The listing builds one solid part. Answer for the finished solid, in the listing's coordinates (mm). A direction names the side the tool comes from. Coordinates: 2 decimals unless noted, no trailing zeros. Write each loop counter-clockwise with the first axis right and the second up, starting at its lowest first coordinate (ties: lowest second). Pieces come first, ordered by that corner, then holes. Notation, with made-up numbers: M 30.5,-31 L 64.5,-31 A22 cw 64.5,-25 Z; hole C 2,-10 d10. An arc over 180 degrees is marked long. Write item = value, one per line. Start each with the question number.
Solid Edge part; units mm, degrees
sketch "Sketch1" plane through (0, 0, 0) normal (0, 0, 1) x (1, 0, 0)
  line L0 (-10.25, -8) -> (10.25, -8)
  line L1 (10.25, -8) -> (10.25, 8)
  line L2 (10.25, 8) -> (-10.25, 8)
  line L3 (-10.25, 8) -> (-10.25, -8)
  dimension "D1" = 10.25
  dimension "D2" = 10.25
extrude "Protrusion1" add sketch "Sketch1" along normal blind 1.6
sketch "Sketch2" plane through (0, 0, 1.6) normal (0, 0, 1) x (1, 0, 0)
  circle A0 centre (-8, 5.8) radius 1.4
  circle A1 centre (8, 5.8) radius 1.4
extrude "Cutout1" cut sketch "Sketch2" against normal through all
sketch "Sketch3" plane through (0, 0, 1.6) normal (0, 0, 1) x (1, 0, 0)
  line L0 (-10.25, -3.5) -> (10.25, -3.5)
  line L1 (10.25, -3.5) -> (10.25, 4)
  line L2 (6.25, 4) -> (10.25, 4)
  line L3 (6.25, 5) -> (6.25, 4)
  line L4 (3.5, 5) -> (6.25, 5)
  line L5 (3.5, 8) -> (3.5, 5)
  line L6 (3.5, 8) -> (-3.5, 8)
  line L7 (-3.5, 8) -> (-3.5, 5)
  line L8 (-3.5, 5) -> (-6.25, 5)
  line L9 (-6.25, 5) -> (-6.25, 4)
  line L10 (-6.25, 4) -> (-10.25, 4)
  line L11 (-10.25, 4) -> (-10.25, -3.5)
  dimension "D1" = 3.5
  dimension "D2" = 3.5
  dimension "D3" = 10.25
  dimension "D4" = 6.25
  dimension "D5" = 10.25
  dimension "D6" = 3.5
  dimension "D7" = 6.25
extrude "Extrusionsausprägung_2" add sketch "Sketch3" along normal blind 1.5
sketch "Sketch4" plane through (0, -5.75, 1.6) normal (0, 0, 1) x (1, 0, 0)
  circle A0 centre (-8.75, -0.75) radius 0.5
  circle A1 centre (-6.25, -0.75) radius 0.5
  circle A2 centre (-3.75, -0.75) radius 0.5
  circle A3 centre (-1.25, -0.75) radius 0.5
  circle A4 centre (1.25, -0.75) radius 0.5
  circle A5 centre (3.75, -0.75) radius 0.5
  circle A6 centre (6.25, -0.75) radius 0.5
  circle A7 centre (8.75, -0.75) radius 0.5
  dimension "D1" = 8.75
extrude "Cutout2" cut sketch "Sketch4" against normal through all
1. The part is cut by section B-B, the plane y = 5.8. Write down the section's boundary in (x, z), and give its area (3 significant figures).
2. Straight lines are drawn through the part: L1, parallel to Y at x = -3.75, z = 0.8; L2, parallel to Z at x = 7.75, y = -4; L3, parallel to Y at x = 4.75, z = 2.6. For each, find the intervals that lie inside material, in ascending order. Write a range as [from, to].
3. For a pull along Y with two mould halves and no side action, classify faces 1 (the face through (3.35, -6.8, 0.81)), 2 (the face through (0, 0, 0)), 3 (the face through (8, 4, 2)) as pulls with the +Y half, pulls with the -Y half, needs draft (parallel to the pull), parting line crosses it, or undercut.
4. Each of these flat-tipped pins is pushed along its axis until it touches: pin 1 (0.8 mm diameter, centred on y = 6.5, z = 2.5, fed in from +X); pin 2 (3.5 mm diameter, centred on x = -3.5, y = -5.5, fed in from +Z). Where does it stop, or does it pass through?
5. For faces 4 (the face through (-6.65, -6.8, 0.81)), 5 (the face through (-3.5, 7, 2)), 6 (the face through (0, -6, 1.6)), 7 (the face through (6.25, 4.5, 2.3)), determine the directions among +Z, -Z, +X, -X, +Y, -Y from which every point of the face is accessible in a straight line to the end or side of a thin tool.
6. The part is cut by section D-D, the plane x = 4.5. Write down the section's boundary in (y, z).
7. The part is cut by section C-C, the plane z = 0.4. Count the separate pieces of the cut face and the enclosed holes in it, and give its area (3 significant figures).
8. The part is cut by section A-A, the plane x = -3.75. Write down the section's boundary in (y, z).
Solution:
q1.outline = M -10.25,0 L -9.4,0 L -9.4,1.6 L -10.25,1.6 Z; M -6.6,0 L 6.6,0 L 6.6,1.6 L 3.5,1.6 L 3.5,3.1 L -3.5,3.1 L -3.5,1.6 L -6.6,1.6 Z; M 9.4,0 L 10.25,0 L 10.25,1.6 L 9.4,1.6 Z
q1.area = 34.3 mm^2
q2.L1 = [-8, -7], [-6, 8]
q2.L2 = [0, 1.6]
q2.L3 = [-3.5, 5]
q3.face_1 = undercut
q3.face_2 = needs draft
q3.face_3 = pulls with the +Y half
q4.pin_1 = 3.5
q4.pin_2 = 1.6
q5.face_4 = +Z, -Z
q5.face_5 = +Z, -X, +Y
q5.face_6 = +Z, +X, -X, -Y
q5.face_7 = +Z, +X, +Y
q6.outline = M -8,0 L 8,0 L 8,1.6 L 5,1.6 L 5,3.1 L -3.5,3.1 L -3.5,1.6 L -8,1.6 Z
q7.separate_pieces = 1
q7.enclosed_holes = 10
q7.area = 309 mm^2
q8.outline = M -8,0 L -7,0 L -7,1.6 L -8,1.6 Z; M -6,0 L 8,0 L 8,1.6 L 5,1.6 L 5,3.1 L -3.5,3.1 L -3.5,1.6 L -6,1.6 Z
